Source: CAD feature listing. Evaluate the final solid. Frame: model axes, mm. Give positions to 0.01 mm unless a question says otherwise; leave off trailing zeros. Loops run counter-clockwise (first coordinate to the right, second up) from the corner with the lowest first, then second, coordinate; pieces in that order, holes last. Notation, with made-up numbers: M 37,-22 L 52,-22 A3 cw 52,-18 Z; hole C 33.5,-31 d4. An arc over 180 degrees is marked long. Answer in a Markdown table with one row per item.
```python
from build123d import *

# Parameters (mm, degrees)
SKETCH1_R           = 3
BOSS_EXTRUDE1_DEPTH = 4.7
FILLET1_R           = 0.5


with BuildPart() as part:
    # Sketch1 → Boss-Extrude1 (new body)
    with BuildSketch(Plane.XY):
        Polygon((-2.740345561, 4.768700683), (-5.499988715, 0.011141471), (-2.759643154, -4.757559213), (2.740345561, -4.768700683), (5.499988715, -0.011141471), (2.759643154, 4.757559213), align=None)
        Circle(SKETCH1_R, mode=Mode.SUBTRACT)
    extrude(amount=BOSS_EXTRUDE1_DEPTH)

    # Fillet1
    fillet1_edges = [part.edges().sort_by_distance(p)[0] for p in [
        (-4.129815935, -2.373208871, 4.7),
        (2.759643154, 4.757559213, 2.35),
        (5.499988715, -0.011141471, 2.35),
        (2.740345561, -4.768700683, 2.35),
        (-2.759643154, -4.757559213, 2.35),
        (-5.499988715, 0.011141471, 2.35),
        (-2.740345561, 4.768700683, 2.35),
        (-0.009648797, -4.763129948, 4.7),
        (4.120167138, -2.389921077, 4.7),
        (-3, 0, 0),
        (-3, 0, 4.7),
        (4.129815935, 2.373208871, 4.7),
        (0.009648797, 4.763129948, 4.7),
        (4.129815935, 2.373208871, 0),
        (4.120167138, -2.389921077, 0),
        (-0.009648797, -4.763129948, 0),
        (-4.120167138, 2.389921077, 4.7),
        (-4.129815935, -2.373208871, 0),
        (-4.120167138, 2.389921077, 0),
        (0.009648797, 4.763129948, 0),
    ]]
    fillet(fillet1_edges, radius=FILLET1_R)


solid = part.part
```
Q1. Mould query, pull axis Y, two halves, no side actions, for faces 1 (the cylindrical face through (-4.01, 2.29, 0.15)), 2 (the cylindrical face through (-3, 0, 2)), 3 (the flat face through (3, 3, 4.7)), 4 (the cylindrical face through (4.01, -2.29, 4.55)). Classes: +Y half, -Y half, draft (parallel to the pull), parting line (faces both ways), or undercut.
Values follow:
| item | result |
|---|---|
| face 1 | +Y half |
| face 2 | undercut |
| face 3 | draft |
| face 4 | -Y half |
Q2. Ray query, probe 1 along Y at (x, z) = (-0.25, 1.65); probe 2 along X at (y, z) = (-2.5, 1.7); probe 3 along Y at (x, z) = (-2, 2.55). Return the intervals inside material, ascending. Write a range as from..to.
Values follow:
| item | result |
|---|---|
| probe 1 | -4.76..-2.99, 2.99..4.76 |
| probe 2 | -4.06..-1.66, 1.66..4.06 |
| probe 3 | -4.76..-2.24, 2.24..4.77 |
Q3. Contact query for a flat-ended pin moving along its axis: pin 1 Ø3.5 at (x, y) = (0, 0) entering from +Z. Output: stop coordinate, or through.
Values follow:
| item | result |
|---|---|
| pin 1 | through |
Q4. Section query A-A (z = 1.75). Output: boundary loops of the cut face in (x, y).
Values follow:
| item | result |
|---|---|
| outline | M -5.36,-0.24 L -2.9,-4.51 A0.5 ccw -2.47,-4.76 L 2.45,-4.77 A0.5 ccw 2.89,-4.52 L 5.36,-0.26 A0.5 ccw 5.36,0.24 L 2.9,4.51 A0.5 ccw 2.47,4.76 L -2.45,4.77 A0.5 ccw -2.89,4.52 L -5.36,0.26 A0.5 ccw Z; hole C 0,0 d6 |
